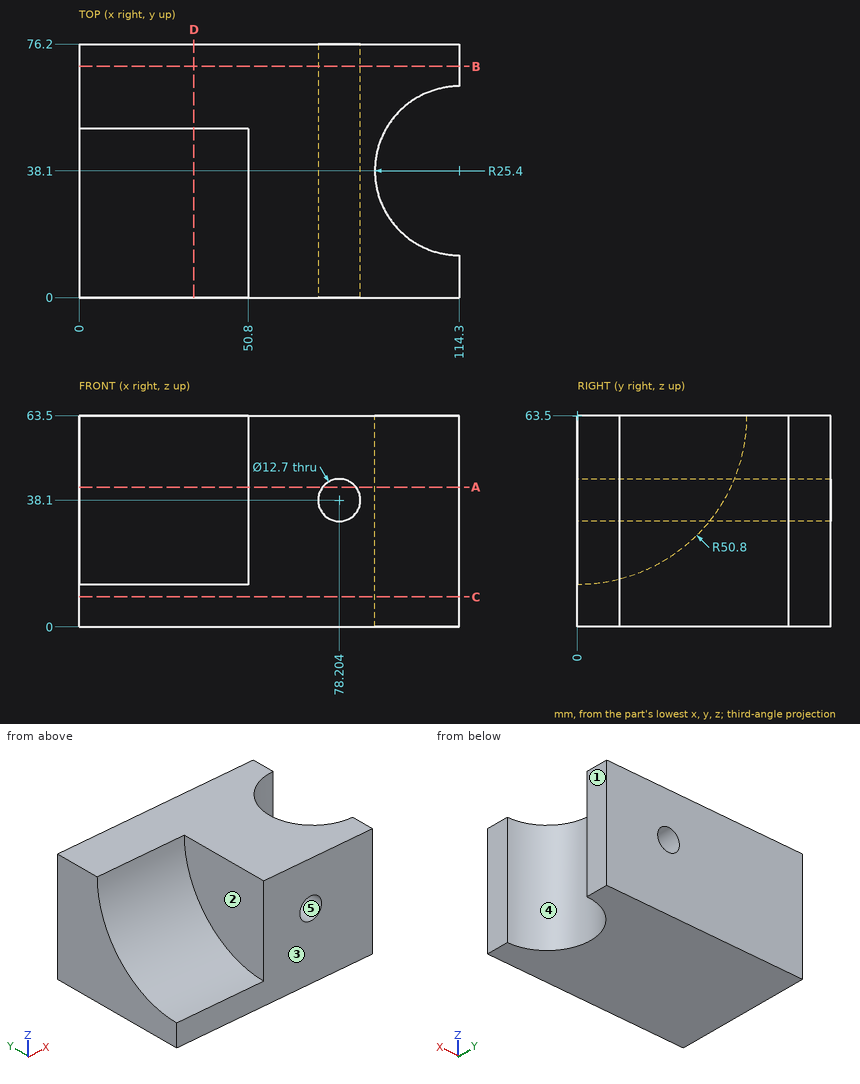
Design review of the part shown in the three views and the two pictorial views. Dimensions are in mm from the part's minimum x, y and z. A direction names the side the tool comes from. Give positions to 0.01 mm unless a question says otherwise; leave off trailing zeros. Write each loop counter-clockwise with the first axis right and the second up, starting at its lowest first coordinate (ties: lowest second). Pieces come first, ordered by that corner, then holes. Notation, with made-up numbers: M 39.25,25 L 75.25,25 A32 cw 75.25,63 Z; hole C 12.25,75.5 d6. An arc over 180 degrees is marked long. Answer in a Markdown table with one row per item.
Item 1: For P1, Ø4, axis at x = 13, y = 28.5, coming from the +Z side (1 decimal); P2, Ø1.5, axis at x = 85, y = 63.5, coming from the -Z side; P3, Ø1, axis at x = 28, y = 20, coming from the +Z side, all flat-tipped, find the tip position at first contact; note any pin that passes through.
Check sheet entries:
| item | result |
|---|---|
| P1 | z = 22.9 |
| P2 | z = 0 |
| P3 | z = 17.02 |
Item 2: For line 1 along Y through (x, z) = (107, 28); line 2 along X through (y, z) = (35, 38.5); line 3 along X through (y, z) = (17, 38) (1 decimal), list the stretches that pass through material, from the lowest coordinate up.
Check sheet entries:
| item | result |
|---|---|
| line 1 | 0 to 13.77, 62.43 to 76.2 |
| line 2 | 50.8 to 71.87, 84.54 to 89.09 |
| line 3 | 50.8 to 71.9, 84.6 to 100.2 |
Item 3: Add section C-C on z = 9. Give the boundary of the cut face in (x, y), plus the area to 3 significant figures.
Check sheet entries:
| item | result |
|---|---|
| outline | M 0,0 L 114.3,0 L 114.3,12.7 A25.4 cw 114.3,63.5 L 114.3,76.2 L 0,76.2 Z |
| area | 7,700 mm2 |
Item 4: Add section A-A on z = 42. Give the boundary of the cut face in (x, y), plus the area to 3 significant figures.
Check sheet entries:
| item | result |
|---|---|
| outline | M 0,46.03 L 50.8,46.03 L 50.8,0 L 73.19,0 L 73.19,76.2 L 0,76.2 Z; M 83.22,0 L 114.3,0 L 114.3,12.7 A25.4 cw 114.3,63.5 L 114.3,76.2 L 83.22,76.2 Z |
| area | 4,590 mm2 |
Item 5: Draft analysis for pull direction X (two halves, no side actions). For the marked faces 3, 4 and 5, state which applies: +X half, -X half, draft (parallel to the pull), parting line (faces both ways), or undercut.
Check sheet entries:
| item | result |
|---|---|
| face 3 | draft |
| face 4 | +X half |
| face 5 | undercut |
Item 6: Tool access review of the marked faces 1 and 2: name each direction out of +Z, -Z, +X, -X, +Y, -Y from which nothing blocks a thin tool from reaching the whole face with its end or side.
Check sheet entries:
| item | result |
|---|---|
| face 1 | +Z, -Z, +X, +Y, -Y |
| face 2 | +Z, -X, -Y |
Item 7: Add section D-D on x = 34.5. Give the boundary of the cut face in (y, z), plus the area to 3 significant figures.
Check sheet entries:
| item | result |
|---|---|
| outline | M 0,0 L 76.2,0 L 76.2,63.5 L 50.8,63.5 A50.8 cw 0,12.7 Z |
| area | 2,810 mm2 |
Item 8: Add section B-B on y = 69.5. Give the boundary of the cut face in (x, z).
Check sheet entries:
| item | result |
|---|---|
| outline | M 0,0 L 114.3,0 L 114.3,63.5 L 0,63.5 Z; hole C 78.2,38.1 d12.7 |
